```python
from build123d import *

# Parameters (mm, degrees)
SKETCH1_R               = 12.5
SKETCH1_R_2             = 4.5
BOSS_EXTRUDE1_DEPTH     = 10
SKETCH2_W               = 9.983536535
SKETCH2_H               = 1
CUT_EXTRUDE1_DEPTH      = 21.310096012
CUT_EXTRUDE2_DEPTH      = 21.310096012
CUT_EXTRUDE2_DEPTH_BACK = 21.310096012
SKETCH3_R               = 2
CUT_EXTRUDE3_REACH      = 25.351
SKETCH4_R               = 3.6
CUT_EXTRUDE4_REACH      = 25.351
CUT_EXTRUDE4_END_RADIUS = 12.5


with BuildPart() as part:
    # Sketch1 → Boss-Extrude1 (new body)
    with BuildSketch(Plane.XY):
        Circle(SKETCH1_R)
        Circle(SKETCH1_R_2, mode=Mode.SUBTRACT)
    extrude(amount=BOSS_EXTRUDE1_DEPTH)

    # Sketch2 → Cut-Extrude1 (cut, through all)
    with BuildSketch(Plane.XY.offset(10)):
        with Locations((8.497672296, 0)):
            Rectangle(SKETCH2_W, SKETCH2_H)
    extrude(amount=-CUT_EXTRUDE1_DEPTH, mode=Mode.SUBTRACT)

    # Sketch3 → Cut-Extrude2 (cut, two sides: drawn at the far end of the back side and taken through both)
    with BuildSketch(Plane(origin=(0, 0, 0), x_dir=(1, 0, 0), z_dir=(0, 1, 0)).offset(-CUT_EXTRUDE2_DEPTH_BACK)):
        with Locations(Location((8.481065976, -5, 0), (0, 0, 270))):
            Circle(SKETCH3_R)
    extrude(amount=CUT_EXTRUDE2_DEPTH + CUT_EXTRUDE2_DEPTH_BACK, mode=Mode.SUBTRACT)

    # Sketch4 → Cut-Extrude3 (cut, up to next)
    with BuildSketch(Plane(origin=(0, 4.5, 0), x_dir=(1, 0, 0), z_dir=(0, 1, 0)), mode=Mode.PRIVATE) as cut_extrude3_sk1:
        with Locations((8.481065976, -5)):
            Circle(SKETCH4_R)
    cut_extrude3_tool1 = extrude(cut_extrude3_sk1.sketch, amount=CUT_EXTRUDE3_REACH, mode=Mode.PRIVATE) & part.part
    add(cut_extrude3_tool1.solids().sort_by_distance((8.481066, 4.5, 5))[0], mode=Mode.SUBTRACT)

    # Cut-Extrude4: up to this cylinder (the profile starts inside it)
    cut_extrude4_end = Plane(origin=(0, 0, 5), z_dir=(0, 0, -1)) * Cylinder(CUT_EXTRUDE4_END_RADIUS, 76.702, mode=Mode.PRIVATE)
    # Sketch5 → Cut-Extrude4 (cut, up to the surface)
    with BuildSketch(Plane(origin=(0, -4.5, 0), x_dir=(1, 0, 0), z_dir=(0, 1, 0)), mode=Mode.PRIVATE) as cut_extrude4_sk1:
        Polygon((8.472706177, -9.099178387), (12.026878694, -7.056828991), (12.035238493, -2.957650604), (8.489425774, -0.900821613), (4.935253257, -2.943171009), (4.926893459, -7.042349396), align=None)
    cut_extrude4_tool1 = extrude(cut_extrude4_sk1.sketch, amount=-CUT_EXTRUDE4_REACH, mode=Mode.PRIVATE) & cut_extrude4_end
    add(cut_extrude4_tool1.solids().sort_by_distance((8.481066, -4.5, 5))[0], mode=Mode.SUBTRACT)


solid = part.part
```
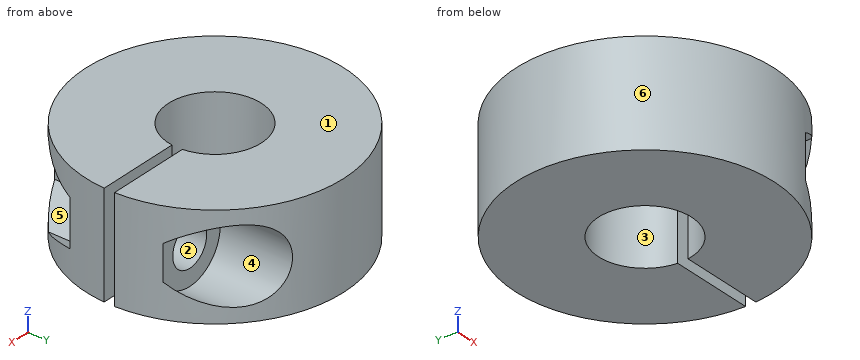
Read the model definition and answer for the solid it produces. Units are mm, in the model's axes. Face numbers are marked on the shaded views. A direction names the side the tool comes from. Give positions to 0.01 mm unless a question says otherwise; leave off trailing zeros. Write each loop counter-clockwise with the first axis right and the second up, starting at its lowest first coordinate (ties: lowest second). Pieces come first, ordered by that corner, then holes. Notation, with made-up numbers: (-13.5, 58) - (6.5, 58) arc R17 cw to (6.5, 89) - close; hole circle Ø11 at (67.5, -5). An arc over 180 degrees is marked (long way). Write item = value, one per line. Start each with the question number.
Item 1: Find section C-C (x = 0). Give the vertices of the cut face in (y, z), then the cut area to 3 significant figures.
Item 2: Find section D-D (z = 5.5). Give the vertices of the cut face in (x, y), then the cut area to 3 significant figures.
Item 3: Each of these flat-tipped pins is pushed along its axis until it touches: P1, Ø1, axis at y = -6, z = 7, coming from the -X side (3 decimals); P2, Ø6, axis at x = -6, z = 8, coming from the -Y side; P3, Ø5, axis at x = 8.48, z = 5, coming from the -Y side. Where does it stop, or does it pass through?
Item 4: Find the intervals of material crossed by probe 1 along Y at (x, z) = (0.25, 4); probe 2 along X at (y, z) = (0, 2.75); probe 3 along X at (y, z) = (-5.5, 1.5), in increasing order. Write a range as [from, to].
Item 5: A tool of negligible diameter and unlimited length cuts with its end or side. For the marked faces 4, 5 and 6, from which of +Z, -Z, +X, -X, +Y, -Y can it reach the whole face along a straight path? Write none if from no direction.
Item 6: Find section B-B (x = 7.5). Give the vertices of the cut face in (y, z).
Item 7: The mould has two halves that part along Z. Classify the marked faces 1, 2 and 3: +Z half, -Z half, draft (parallel to the pull), parting line (faces both ways), or undercut.
Item 8: Find section A-A (y = -1.75). Give the vertices of the cut face in (x, z).
Response:
q1.outline = (-12.5, 0) - (-4.5, 0) - (-4.5, 10) - (-12.5, 10) - close; (4.5, 0) - (12.5, 0) - (12.5, 10) - (4.5, 10) - close
q1.area = 160 mm²
q2.outline = (4.47, -0.5) arc R4.5 cw (long way) to (4.47, 0.5) - (6.54, 0.5) - (6.54, 4.5) - (4.92, 4.5) - (4.92, 11.49) arc R12.5 ccw (long way) to (4.93, -11.49) - (4.93, -4.5) - (6.54, -4.5) - (6.54, -0.5) - close; (10.42, -4.5) - (11.66, -4.5) arc R12.5 ccw to (12.49, -0.5) - (10.42, -0.5) - close; (10.42, 0.5) - (12.49, 0.5) arc R12.5 ccw to (11.66, 4.5) - (10.42, 4.5) - close
q2.area = 328 mm²
q3.P1 = -11.225
q3.P2 = -12.13
q3.P3 = -4.5
q4.probe_1 = [-12.5, -4.49], [4.49, 12.5]
q4.probe_2 = [-12.5, -4.5]
q4.probe_3 = [-11.22, 7.45], [9.52, 11.22]
q5.face_4 = +Y
q5.face_5 = -Y
q5.face_6 = +Z, -Z
q6.outline = (-10, 0) - (-0.5, 0) - (-0.5, 3.26) - (-4.5, 3.26) - (-4.5, 1.47) - (-10, 1.47) - close; (-10, 8.53) - (-4.5, 8.53) - (-4.5, 6.74) - (-0.5, 6.74) - (-0.5, 10) - (-10, 10) - close; (0.5, 0) - (10, 0) - (10, 1.54) - (4.5, 1.54) - (4.5, 3.26) - (0.5, 3.26) - close; (0.5, 6.74) - (4.5, 6.74) - (4.5, 8.46) - (10, 8.46) - (10, 10) - (0.5, 10) - close
q7.face_1 = +Z half
q7.face_2 = undercut
q7.face_3 = draft
q8.outline = (-12.38, 0) - (-4.15, 0) - (-4.15, 10) - (-12.38, 10) - close; (4.15, 0) - (12.38, 0) - (12.38, 10) - (4.15, 10) - close; hole circle Ø4 at (8.48, 5)
